from build123d import *

# Parameters (mm, degrees)
SKETCH1_W           = 40.3
SKETCH1_H           = 27
BOSS_EXTRUDE1_DEPTH = 20
SKETCH2_W           = 40.3
SKETCH2_H           = 5.05
SKETCH2_H_2         = 9.9
BOSS_EXTRUDE2_DEPTH = 2.7
SKETCH3_W           = 39.7
SKETCH3_H           = 20
BOSS_EXTRUDE3_DEPTH = 10.2
BOSS_EXTRUDE4_DEPTH = 4
SKETCH5_W           = 3.501362038
SKETCH5_H           = 11.379426624
BOSS_EXTRUDE5_DEPTH = 4


with BuildPart() as part:
    # Sketch1 → Boss-Extrude1 (new body)
    with BuildSketch(Plane(origin=(0, 0, 0), x_dir=(1, 0, 0), z_dir=(0, 1, 0))):
        Rectangle(SKETCH1_W, SKETCH1_H)
    extrude(amount=BOSS_EXTRUDE1_DEPTH)

    # Sketch2 → Boss-Extrude2 (add)
    with BuildSketch(Plane.XY.offset(13.5)):
        with Locations((0, 2.525)):
            Rectangle(SKETCH2_W, SKETCH2_H)
        with BuildLine():
            Line((-20.15, 0), (-20.15, 5.05))
            Line((-20.15, 5.05), (-21.75, 5.05))
            ThreePointArc((-21.75, 5.05), (-22.82883539, 3.12883539), (-25.030776406, 3.05))
            Line((-25.030776406, 3.05), (-27.15, 3.05))
            Line((-27.15, 3.05), (-27.15, 0))
            Line((-27.15, 0), (-20.15, 0))
        make_face()
        with Locations((0, 10)):
            Rectangle(SKETCH2_W, SKETCH2_H_2)
        with BuildLine():
            Line((-20.15, 5.05), (-20.15, 14.95))
            Line((-20.15, 14.95), (-21.75, 14.95))
            ThreePointArc((-21.75, 14.95), (-22.409009742, 13.359009742), (-24, 12.7))
            Line((-24, 12.7), (-24, 7.3))
            ThreePointArc((-24, 7.3), (-22.409009742, 6.640990258), (-21.75, 5.05))
            Line((-21.75, 5.05), (-20.15, 5.05))
        make_face()
        with BuildLine():
            Line((-25.030776406, 12.95), (-27.15, 12.95))
            Line((-27.15, 12.95), (-27.15, 7.05))
            Line((-27.15, 7.05), (-25.030776406, 7.05))
            ThreePointArc((-25.030776406, 7.05), (-24.530330086, 7.236606961), (-24, 7.3))
            Line((-24, 7.3), (-24, 12.7))
            ThreePointArc((-24, 12.7), (-24.530330086, 12.763393039), (-25.030776406, 12.95))
        make_face()
        with Locations((0, 17.475)):
            Rectangle(SKETCH2_W, SKETCH2_H)
        with BuildLine():
            Line((-20.15, 14.95), (-20.15, 20))
            Line((-20.15, 20), (-27.15, 20))
            Line((-27.15, 20), (-27.15, 16.95))
            Line((-27.15, 16.95), (-25.030776406, 16.95))
            ThreePointArc((-25.030776406, 16.95), (-22.82883539, 16.87116461), (-21.75, 14.95))
            Line((-21.75, 14.95), (-20.15, 14.95))
        make_face()
        with BuildLine():
            Line((27.15, 20), (20.15, 20))
            Line((20.15, 20), (20.15, 14.95))
            Line((20.15, 14.95), (21.75, 14.95))
            ThreePointArc((21.75, 14.95), (22.82883539, 16.87116461), (25.030776406, 16.95))
            Line((25.030776406, 16.95), (27.15, 16.95))
            Line((27.15, 16.95), (27.15, 20))
        make_face()
        with BuildLine():
            Line((27.15, 7.05), (27.15, 12.95))
            Line((27.15, 12.95), (25.030776406, 12.95))
            ThreePointArc((25.030776406, 12.95), (24.530330086, 12.763393039), (24, 12.7))
            Line((24, 12.7), (24, 7.3))
            ThreePointArc((24, 7.3), (24.530330086, 7.236606961), (25.030776406, 7.05))
            Line((25.030776406, 7.05), (27.15, 7.05))
        make_face()
        with BuildLine():
            Line((21.75, 5.05), (20.15, 5.05))
            Line((20.15, 5.05), (20.15, 0))
            Line((20.15, 0), (27.15, 0))
            Line((27.15, 0), (27.15, 3.05))
            Line((27.15, 3.05), (25.030776406, 3.05))
            ThreePointArc((25.030776406, 3.05), (22.82883539, 3.12883539), (21.75, 5.05))
        make_face()
        with BuildLine():
            Line((21.75, 14.95), (20.15, 14.95))
            Line((20.15, 14.95), (20.15, 5.05))
            Line((20.15, 5.05), (21.75, 5.05))
            ThreePointArc((21.75, 5.05), (22.409009742, 6.640990258), (24, 7.3))
            Line((24, 7.3), (24, 12.7))
            ThreePointArc((24, 12.7), (22.409009742, 13.359009742), (21.75, 14.95))
        make_face()
    extrude(amount=BOSS_EXTRUDE2_DEPTH)

    # Sketch3 → Boss-Extrude3 (add)
    with BuildSketch(Plane.XY.offset(16.2)):
        with Locations((0, 10)):
            Rectangle(SKETCH3_W, SKETCH3_H)
    extrude(amount=BOSS_EXTRUDE3_DEPTH)

    # Sketch4 → Boss-Extrude4 (add)
    with BuildSketch(Plane.XY.offset(26.4)):
        with BuildLine():
            ThreePointArc((-6.85, 10), (-9.8, 12.95), (-12.75, 10))
            Line((-12.75, 10), (-6.85, 10))
        make_face()
        with BuildLine():
            Line((-6.85, 10), (-12.75, 10))
            ThreePointArc((-12.75, 10), (-9.8, 7.05), (-6.85, 10))
        make_face()
    extrude(amount=BOSS_EXTRUDE4_DEPTH)

    # Sketch5 → Boss-Extrude5 (add)
    with BuildSketch(Plane.ZY.offset(20.15)):
        with Locations((-8.667769888, 10)):
            Rectangle(SKETCH5_W, SKETCH5_H)
    extrude(amount=BOSS_EXTRUDE5_DEPTH)


solid = part.part
Check sheet for the modelled part. Datum: model origin and axes. Units: mm. A direction names the side the tool comes from. Give positions to 0.01 mm unless a question says otherwise; leave off trailing zeros. Loops run counter-clockwise (first coordinate to the right, second up) from the corner with the lowest first, then second, coordinate; pieces in that order, holes last. Notation, with made-up numbers: M 48.25,-7.75 L 101.25,-7.75 A16 cw 101.25,9.25 Z; hole C 18,83.25 d1. An arc over 180 degrees is marked long. Use a Markdown table: item, result. Add a question column.
Q1. Tool access check on faces 1 (the flat face through (19.85, 10, 21)), 2 (the flat face through (-22, 15.69, -9)), 3 (the flat face through (-26, 16.95, 15)). Record the directions out of +Z, -Z, +X, -X, +Y, -Y that give a thin tool (end or side, any length) a straight path to the whole face; none if there is none.
Q2. Sectioned sample at D-D, the plane x = 21. Record the cut outline in (y, z), then the cut area to 3 significant figures.
Q3. Go/stop test with flat-tipped pins: pin 1 (12 mm diameter, centred on y = 8.5, z = 24, fed in from +X); pin 2 (10 mm diameter, centred on x = -2, y = 12, fed in from +Z); pin 3 (10 mm diameter, centred on y = 7.5, z = -5.5, fed in from +X); pin 4 (1.7 mm diameter, centred on x = -26, z = 14.5, fed in from -Y). Record where each tip stops, or that it passes through.
Q4. Sectioned sample at B-B, the plane x = -9.8. Record the cut outline in (y, z), then the cut area to 3 significant figures.
Q5. Mould release check, pull along Z, two halves, no side actions. Record for faces 4 (the flat face through (-23, 10, 13.5)), 5 (the flat face through (-20.15, 10, 0)), 6 (the flat face through (-26, 7.05, 15)), 7 (the flat face through (-10, 10, 30.4)): pulls with the +Z half, pulls with the -Z half, needs draft (parallel to the pull), parting line crosses it, or undercut.
Q6. Sectioned sample at A-A, the plane y = 10. Record the cut outline in (x, z), then the cut area to 3 significant figures.
Q7. Sectioned sample at C-C, the plane z = 25. Record the cut outline in (x, y).
Q8. Scan lines: line 1 along X through (y, z) = (4, -3.5); line 2 along Z through (x, y) = (-6, 15); line 3 along Z through (x, y) = (-20.5, 4.25). Record each from-to range of solid material in increasing order. Write a range as [from, to].
Verdict:
| question | item | result |
|---|---|---|
| 1 | face 1 | +Z, +X, +Y, -Y |
| 1 | face 2 | -Z, -X, +Y |
| 1 | face 3 | +Z, -Z, -X |
| 2 | outline | M 0,13.5 L 20,13.5 L 20,16.2 L 0,16.2 Z |
| 2 | area | 54.0 mm^2 |
| 3 | pin 1 | x = 19.85 |
| 3 | pin 2 | z = 26.4 |
| 3 | pin 3 | x = 20.15 |
| 3 | pin 4 | y = 0 |
| 4 | outline | M 0,-13.5 L 20,-13.5 L 20,26.4 L 12.95,26.4 L 12.95,30.4 L 7.05,30.4 L 7.05,26.4 L 0,26.4 Z |
| 4 | area | 822 mm^2 |
| 5 | face 4 | undercut |
| 5 | face 5 | undercut |
| 5 | face 6 | needs draft |
| 5 | face 7 | pulls with the +Z half |
| 6 | outline | M -27.15,13.5 L -20.15,13.5 L -20.15,-6.92 L -24.15,-6.92 L -24.15,-10.42 L -20.15,-10.42 L -20.15,-13.5 L 20.15,-13.5 L 20.15,13.5 L 27.15,13.5 L 27.15,16.2 L 19.85,16.2 L 19.85,26.4 L -6.85,26.4 L -6.85,30.4 L -12.75,30.4 L -12.75,26.4 L -19.85,26.4 L -19.85,16.2 L -27.15,16.2 Z |
| 6 | area | 1,680 mm^2 |
| 7 | outline | M -19.85,0 L 19.85,0 L 19.85,20 L -19.85,20 Z |
| 8 | line 1 | [-20.15, 20.15] |
| 8 | line 2 | [-13.5, 26.4] |
| 8 | line 3 | [13.5, 16.2] |
